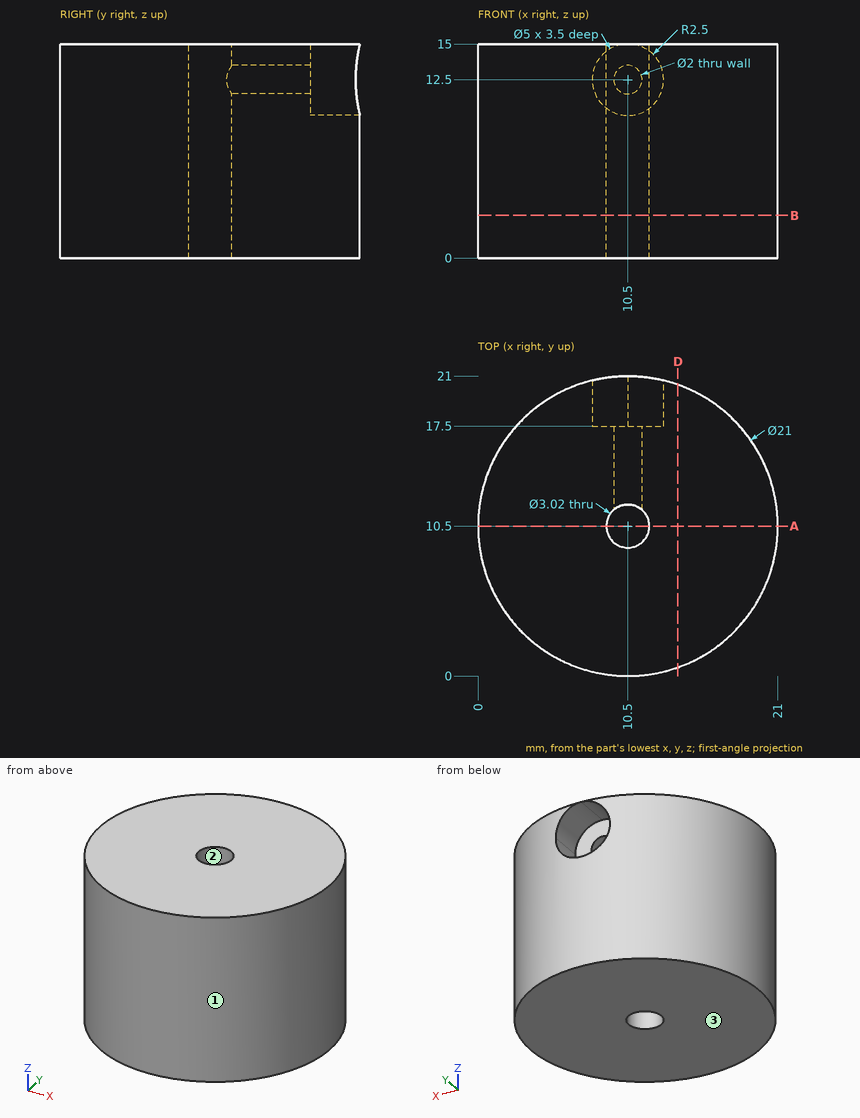
Study the drawing (mm; zero at the part's minimum x, y, z) and answer. Coordinates: 2 decimals unless noted, no trailing zeros. Write each loop counter-clockwise with the first axis right and the second up, starting at its lowest first coordinate (ties: lowest second). Pieces come first, ordered by that corner, then holes. Notation, with made-up numbers: (48, 37) - (91, 37) arc R20 cw to (91, 47) - close; hole circle Ø4 at (-9.5, 25). An arc over 180 degrees is marked (long way). One line per item, written item: value.
1) Find section B-B (z = 3). Give the vertices of the cut face in (x, y).
Geometry check:
outline: circle Ø21 at (10.5, 10.5); hole circle Ø3.02 at (10.5, 10.5)
2) Consider line 1 along Y through (x, z) = (10.5, 2.75); line 2 along Z through (x, y) = (10.5, 13.85); line 3 along Y through (x, z) = (10.5, 12). Determine where each line is inside the solid, lowest interval first. Write a range as from..to.
Geometry check:
line 1: y = 0..8.99, 12.01..21
line 2: z = 0..11.5, 13.5..15
line 3: y = 0..8.99
3) Find section D-D (x = 14). Give the vertices of the cut face in (y, z), and give its area (3 significant figures).
Geometry check:
outline: (0.6, 0) - (20.4, 0) - (20.4, 15) - (0.6, 15) - close
area: 297 mm2
4) Find section A-A (y = 10.5). Give the vertices of the cut face in (x, z), and give its area (3 significant figures).
Geometry check:
outline: (0, 0) - (8.99, 0) - (8.99, 15) - (0, 15) - close; (12.01, 0) - (21, 0) - (21, 15) - (12.01, 15) - close
area: 270 mm2
5) Each of these flat-tipped pins is pushed along its axis until it touches: pin 1 Ø1 at (x, z) = (12, 2.5) entering from +Y; pin 2 Ø2.5 at (x, z) = (10, 12.5) entering from +Y; pin 3 Ø3 at (x, z) = (17, 1.5) entering from +Y; pin 4 Ø3.5 at (x, y) = (10.5, 10.5) entering from -Z. Where does it stop, or does it pass through?
Geometry check:
pin 1: stops at y = 20.95
pin 2: stops at y = 17.5
pin 3: stops at y = 19.73
pin 4: stops at z = 0
6) For a pull along Y with two mould halves and no side action, classify the marked faces 1, 2 and 3 as pulls with the +Y half, pulls with the -Y half, needs draft (parallel to the pull), parting line crosses it, or undercut.
Geometry check:
face 1: parting line crosses it
face 2: undercut
face 3: needs draft
